Verification items for the finished model (mm, model axes). A direction names the side the tool comes from. Give positions to 0.01 mm unless a question says otherwise; leave off trailing zeros. Loops run counter-clockwise (first coordinate to the right, second up) from the corner with the lowest first, then second, coordinate; pieces in that order, holes last. Notation, with made-up numbers: (52, 73) - (76, 73) arc R15 ccw to (76, 77) - close; hole circle Ø8 at (-30.75, 79). An arc over 180 degrees is marked (long way). One line per question, with ' | ' between items. Start each with the question number.
1. Thickness scan on line 1 along Y through (x, z) = (-28.5, 4); line 2 along Y through (x, z) = (-24, 20.75); line 3 along X through (y, z) = (29, 2). Record the ranges inside material, lowest first. Write a range as from..to.
2. Section check C-C, the plane y = 73. Enter the section's corners in (x, z), then the cut area to 3 significant figures.
3. Section check B-B, the plane x = 0. Enter the section's corners in (y, z).
4. Section check A-A, the plane z = 23. Enter the section's corners in (x, y).
5. Section check D-D, the plane z = 1.75. Enter the section's corners in (x, y).
6. Mould release check, pull along Y, two halves, no side actions. Record for faces 1 (the face through (-22, 95, 10)), 2 (the face through (0.65, 2.53, 12.07)), 3 (the face through (-25.5, 70, 3)), 4 (the face through (-36, 48, 5)): +Y half, -Y half, draft (parallel to the pull), parting line (faces both ways), or undercut.
7. Tool access check on faces 5 (the face through (6, 2, 12)), 6 (the face through (-32, 31.5, 3)), 7 (the face through (-2, 47, 3)). Record the directions out of +Z, -Z, +X, -X, +Y, -Y that give a thin tool (end or side, any length) a straight path to the whole face; none if there is none.
8. Depth check by flat-ended pin: pin 1 Ø12 at (x, z) = (-57, 15.5) entering from -Y; pin 2 Ø1.5 at (y, z) = (44.5, 2) entering from +X; pin 3 Ø5.5 at (y, z) = (71, 2.5) entering from -X; pin 4 Ø4 at (x, y) = (-18, 41) entering from +Z. Enter the tip coordinate at first touch or a pass-through.
from build123d import *

# Parameters (mm, degrees)
BOSS_EXTRUDE1_DEPTH = 5
SKETCH2_W           = 13
SKETCH2_H           = 13
CUT_EXTRUDE1_DEPTH  = 119.11011811
SKETCH5_W           = 76
SKETCH5_H           = 5
BOSS_EXTRUDE3_DEPTH = 20
CUT_EXTRUDE2_DEPTH  = 121.623380818
SKETCH7_R           = 3
CUT_EXTRUDE4_DEPTH  = 121.623380818
SKETCH8_W           = 8
SKETCH8_H           = 85
CUT_EXTRUDE5_DEPTH  = 120.687092036


with BuildPart() as part:
    # Sketch1 → Boss-Extrude1 (new body)
    with BuildSketch(Plane.XY):
        Polygon((-70, 0), (6, 0), (6, 95), (-51, 95), (-70, 47), align=None)
    extrude(amount=BOSS_EXTRUDE1_DEPTH)

    # Sketch2 → Cut-Extrude1 (cut, through all)
    with BuildSketch(Plane.XY.offset(5)):
        with Locations((-32, 70)):
            Rectangle(SKETCH2_W, SKETCH2_H)
        with Locations((-32, 25)):
            Rectangle(SKETCH2_W, SKETCH2_H)
        with Locations((-51, 47.5)):
            Rectangle(SKETCH2_W, SKETCH2_H)
    extrude(amount=-CUT_EXTRUDE1_DEPTH, mode=Mode.SUBTRACT)

    # Sketch5 → Boss-Extrude3 (add)
    with BuildSketch(Plane.XY.offset(5)):
        Polygon((-51, 95), (-52.979166667, 90), (6, 90), (6, 95), align=None)
        with Locations((-32, 2.5)):
            Rectangle(SKETCH5_W, SKETCH5_H)
    extrude(amount=BOSS_EXTRUDE3_DEPTH)

    # Sketch6 → Cut-Extrude2 (cut, through all)
    with BuildSketch(Plane.XZ):
        Polygon((6, 25), (-70, 15), (-70, 25), align=None)
    extrude(amount=-CUT_EXTRUDE2_DEPTH, mode=Mode.SUBTRACT)

    # Sketch7 → Cut-Extrude4 (cut, through all)
    with BuildSketch(Plane(origin=(0, 95, 0), x_dir=(1, 0, 0), z_dir=(0, 1, 0))):
        with Locations(Location((0, -15, 0), (0, 0, 180))):
            Circle(SKETCH7_R)
    extrude(amount=-CUT_EXTRUDE4_DEPTH, mode=Mode.SUBTRACT)

    # Sketch8 → Cut-Extrude5 (cut, through all)
    with BuildSketch(Plane.XY.offset(5)):
        with Locations((2, 47.5)):
            Rectangle(SKETCH8_W, SKETCH8_H)
    extrude(amount=-CUT_EXTRUDE5_DEPTH, mode=Mode.SUBTRACT)


solid = part.part
Results list:
1) line 1: 0..18.5, 31.5..63.5, 76.5..95 | line 2: 0..5, 90..95 | line 3: -70..-38.5, -25.5..-2
2) outline: (-59.71, 0) - (-38.5, 0) - (-38.5, 5) - (-59.71, 5) - close; (-25.5, 0) - (-2, 0) - (-2, 5) - (-25.5, 5) - close | area: 224 mm²
3) outline: (0, 0) - (5, 0) - (5, 12) - (0, 12) - close; (0, 18) - (5, 18) - (5, 24.21) - (0, 24.21) - close; (90, 0) - (95, 0) - (95, 12) - (90, 12) - close; (90, 18) - (95, 18) - (95, 24.21) - (90, 24.21) - close
4) outline: (-9.2, 0) - (6, 0) - (6, 5) - (-9.2, 5) - close; (-9.2, 90) - (6, 90) - (6, 95) - (-9.2, 95) - close
5) outline: (-70, 0) - (6, 0) - (6, 5) - (-2, 5) - (-2, 90) - (6, 90) - (6, 95) - (-51, 95) - (-70, 47) - close; hole (-57.5, 41) - (-44.5, 41) - (-44.5, 54) - (-57.5, 54) - close; hole (-38.5, 18.5) - (-25.5, 18.5) - (-25.5, 31.5) - (-38.5, 31.5) - close; hole (-38.5, 63.5) - (-25.5, 63.5) - (-25.5, 76.5) - (-38.5, 76.5) - close
6) face 1: +Y half | face 2: draft | face 3: undercut | face 4: undercut
7) face 5: +Z, -Z, +X, +Y, -Y | face 6: +Z, -Z | face 7: +Z, -Z, +X
8) pin 1: y = 0 | pin 2: x = -2 | pin 3: x = -61.59 | pin 4: z = 5
